Check sheet for the modelled part. Datum: model origin and axes. Units: mm. Face numbers are marked on the shaded views. A direction names the side the tool comes from. Round coordinates to 2 decimals unless told otherwise and drop trailing zeros. Order: outer loops, then holes, each group sorted by start corner. A loop starts at its lowest first (then second) coordinate and runs counter-clockwise, first axis right, second up.
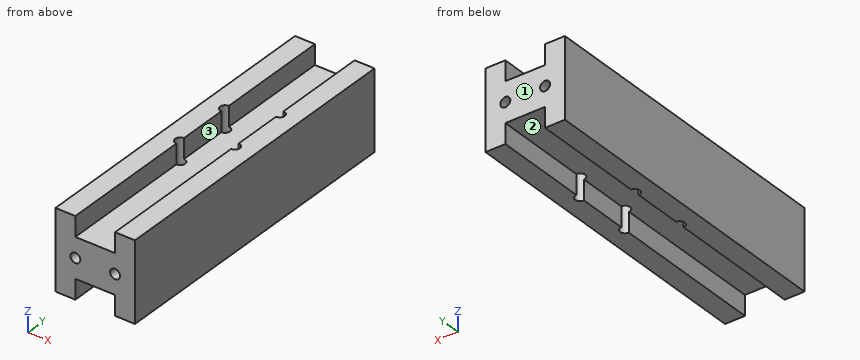
Autodesk Inventor part; units mm, degrees
ref_plane "YZ Plane" through (0, 0, 0) normal (1, 0, 0) x (0, 1, 0)
ref_plane "XZ Plane" through (0, 0, 0) normal (0, 1, 0) x (-1, 0, 0)
ref_plane "XY Plane" through (0, 0, 0) normal (0, 0, 1) x (1, 0, 0)
sketch "Sketch1" plane through (0, 0, 0) normal (0, 1, 0) x (-1, 0, 0)
  line L0 (16.1925, 35.7868) -> (-9.2075, 35.7868)
  line L1 (-9.2075, 35.7868) -> (-9.2075, 10.3868)
  line L2 (-9.2075, 10.3868) -> (16.1925, 10.3868)
  line L3 (16.1925, 10.3868) -> (16.1925, 35.7868)
  point P0 (0, 0)
  dimension "d0" = 25.4
  dimension "d1" = 25.4
extrude "Extrusion1" add sketch "Sketch1" along normal blind 101.6
sketch "Sketch2" plane through (0, 101.6, 0) normal (0, 1, 0) x (1, 0, 0)
  line L0 (-9.8425, -16.7368) -> (2.8575, -16.7368)
  line L1 (2.8575, -16.7368) -> (2.8575, -1.003)
  line L2 (2.8575, -1.003) -> (-9.8425, -1.003)
  line L3 (-9.8425, -1.003) -> (-9.8425, -16.7368)
  line L4 (9.2075, -35.7868) -> (9.2075, -10.3868)
  line L5 (-16.1925, -10.3868) -> (-16.1925, -35.7868)
  line L6 (9.2075, -10.3868) -> (-16.1925, -10.3868)
  point P0 (0, 0)
  dimension "d4" = 6.35
  dimension "d5" = 6.35
  dimension "d6" = 6.35
extrude "Extrusion2" cut sketch "Sketch2" against normal blind 508
sketch "Sketch4" plane through (0, 101.6, 0) normal (0, 1, 0) x (1, 0, 0)
  line L0 (-9.8425, -29.4368) -> (2.8575, -29.4368)
  line L1 (2.8575, -29.4368) -> (2.8575, -45.8861)
  line L2 (2.8575, -45.8861) -> (-9.8425, -45.8861)
  line L3 (-9.8425, -45.8861) -> (-9.8425, -29.4368)
  line L4 (-16.1925, -10.3868) -> (-16.1925, -35.7868)
  line L5 (9.2075, -35.7868) -> (9.2075, -10.3868)
  line L6 (-16.1925, -35.7868) -> (9.2075, -35.7868)
  point P0 (0, 0)
  dimension "d20" = 6.35
  dimension "d21" = 6.35
  dimension "d22" = 6.35
extrude "Extrusion3" cut sketch "Sketch4" against normal blind 508
sketch "Sketch5" plane through (9.2075, 0, 10.3868) normal (0, 0, -1) x (-1, 0, 0)
  line L0 (0, 0) -> (6.35, 0)
  line L1 (0, 0) -> (0, 101.6)
  line L2 (25.4, 0) -> (25.4, 101.6)
  line L3 (19.05, 0) -> (25.4, 0)
  point P0 (9.2075, 0)
  point P1 (19.05, 44.45)
  point P2 (6.35, 50.8)
  dimension "d25" = 50.8
  dimension "d27" = 6.35
  dimension "d28" = 44.45
  dimension "d60" = 19.05
hole "Hole2" at (-9.8425, 44.45, 10.3868) at (2.8575, 50.8, 10.3868) direction (0, 0, 1) diameter 3.175 end through all
sketch "Sketch6" plane through (-16.1925, 0, 10.3868) normal (0, 0, -1) x (-1, 0, 0)
  line L0 (-6.35, 101.6) -> (-6.35, 46.0375)
  line L1 (-25.4, 101.6) -> (-19.05, 101.6)
  line L2 (-25.4, 0) -> (-25.4, 101.6)
  line L3 (-6.35, 101.6) -> (0, 101.6)
  line L4 (0, 0) -> (0, 101.6)
  arc A0 (-19.05, 49.2125) -> (-19.05, 52.3875) centre (-19.05, 50.8) ccw
  arc A1 (-6.35, 46.0375) -> (-6.35, 42.8625) centre (-6.35, 44.45) ccw
  point P0 (-16.1925, 0)
  point P1 (-19.05, 69.85)
  point P2 (-6.35, 63.5)
  dimension "d58" = 6.35
  dimension "d59" = 19.05
  dimension "d61" = 19.05
  dimension "d62" = 19.05
hole "Hole3" at (2.8575, 69.85, 10.3868) at (-9.8425, 63.5, 10.3868) direction (0, 0, 1) diameter 3.175 end through all
sketch "Sketch7" plane through (0, 0, 0) normal (0, -1, 0) x (1, 0, 0)
  line L0 (2.8575, 35.7868) -> (9.2075, 35.7868)
  line L1 (9.2075, 35.7868) -> (9.2075, 10.3868)
  line L2 (-16.1925, 10.3868) -> (-16.1925, 35.7868)
  line L3 (-16.1925, 35.7868) -> (-9.8425, 35.7868)
  point P0 (0, 0)
  point P1 (-9.8425, 23.0868)
  point P2 (2.8575, 23.0868)
  dimension "d47" = 12.7
  dimension "d48" = 6.35
  dimension "d49" = 6.35
  dimension "d50" = 12.7
hole "Hole4" at (-9.8425, 0, 23.0868) at (2.8575, 0, 23.0868) direction (0, 1, 0) diameter 3.175 end through all
properties part number "CarrierBeam"
Item 1: Sectioned sample at B-B (y = 7). Record the cut outline in (x, z) (1 decimal), and give its area (3 significant figures).
Answer:
outline: (-16.2, 10.4) - (-9.8, 10.4) - (-9.8, 16.7) - (2.9, 16.7) - (2.9, 10.4) - (9.2, 10.4) - (9.2, 35.8) - (2.9, 35.8) - (2.9, 29.4) - (-9.8, 29.4) - (-9.8, 35.8) - (-16.2, 35.8) - close; hole circle Ø3.2 at (-9.8, 23.1); hole circle Ø3.2 at (2.9, 23.1)
area: 468 mm2
Item 2: Sectioned sample at C-C (x = -5.5). Record the cut outline in (y, z).
Answer:
outline: (0, 16.74) - (101.6, 16.74) - (101.6, 29.44) - (0, 29.44) - close
Item 3: Access from +Z, -Z, +X, -X, +Y, -Y to the whole of each face (thin tool, end or side, straight path). Record for the marked faces 1, 2 and 3.
Answer:
face 1: +Z, -Z, +X, -X, +Y
face 2: -Z, +Y, -Y
face 3: +Z, +Y, -Y
Item 4: Scan lines: line 1 along Y through (x, z) = (3, 18.25); line 2 along X through (y, z) = (61.5, 14); line 3 along X through (y, z) = (50.8, 29) (1 decimal). Record each from-to range of solid material in increasing order.
Answer:
line 1: y = 0 to 49.22, 52.38 to 68.27, 71.43 to 101.6
line 2: x = -16.19 to -9.84, 2.86 to 9.21
line 3: x = -16.2 to 1.3, 4.4 to 9.2
Item 5: Go/stop test with flat-tipped pins: P1, Ø5, axis at x = 2.86, y = 69.85, coming from the -Z side; P2, Ø4, axis at x = -0.5, y = 17.5, coming from the -Z side; P3, Ø5, axis at x = -1.5, y = 38, coming from the +Z side. Record where each tip stops, or that it passes through.
Answer:
P1: stops at z = 10.39
P2: stops at z = 16.74
P3: stops at z = 29.44
